Could you check a few things on this model? Use its own coordinates, in mm. A direction names the side the tool comes from. Round coordinates to 2 decimals unless told otherwise and drop trailing zeros. Loops run counter-clockwise (first coordinate to the right, second up) from the corner with the lowest first, then second, coordinate; pieces in that order, holes last.
from build123d import *

# Parameters (mm, degrees)
BASE_FLANGE1_DEPTH = 1000
CUT_EXTRUDE2_DEPTH = 1001.734230453
FILLET1_R          = 5


# Sheet-metal steps are written as plain solids
with BuildPart() as part:
    # Sketch1 → Base-Flange1 (new body)
    with BuildSketch(Plane.XY):
        with BuildLine():
            Line((-35.5, -5), (34.7634, -5))
            ThreePointArc((34.7634, -5), (35.284254855, -4.784254855), (35.5, -4.2634))
            Line((35.5, -4.2634), (35.5, 5))
            Line((35.5, 5), (37, 5))
            Line((37, 5), (37, -4.2634))
            ThreePointArc((37, -4.2634), (36.344915027, -5.844915027), (34.7634, -6.5))
            Line((34.7634, -6.5), (-35.5, -6.5))
            Line((-35.5, -6.5), (-35.5, -5))
        make_face()
    extrude(amount=BASE_FLANGE1_DEPTH)

    # Sketch4 → Cut-Extrude2 (cut, through all)
    with BuildSketch(Plane(origin=(0, -5, 0), x_dir=(1, 0, 0), z_dir=(0, 1, 0))):
        with BuildLine():
            ThreePointArc((-20.5, -62.55), (-23.05, -60), (-20.5, -57.45))
            Line((-20.5, -57.45), (-5.5, -57.45))
            ThreePointArc((-5.5, -57.45), (-2.95, -60), (-5.5, -62.55))
            Line((-5.5, -62.55), (-20.5, -62.55))
        make_face()
        with BuildLine():
            ThreePointArc((-20.5, -602.55), (-23.05, -600), (-20.5, -597.45))
            Line((-20.5, -597.45), (-5.5, -597.45))
            ThreePointArc((-5.5, -597.45), (-2.95, -600), (-5.5, -602.55))
            Line((-5.5, -602.55), (-20.5, -602.55))
        make_face()
        with BuildLine():
            ThreePointArc((-5.5, -937.45), (-2.95, -940), (-5.5, -942.55))
            Line((-5.5, -942.55), (-20.5, -942.55))
            ThreePointArc((-20.5, -942.55), (-23.05, -940), (-20.5, -937.45))
            Line((-20.5, -937.45), (-5.5, -937.45))
        make_face()
        with BuildLine():
            ThreePointArc((-5.5, -397.45), (-2.95, -400), (-5.5, -402.55))
            Line((-5.5, -402.55), (-20.5, -402.55))
            ThreePointArc((-20.5, -402.55), (-23.05, -400), (-20.5, -397.45))
            Line((-20.5, -397.45), (-5.5, -397.45))
        make_face()
    extrude(amount=-CUT_EXTRUDE2_DEPTH, mode=Mode.SUBTRACT)

    # Fillet1
    fillet1_edges = [part.edges().sort_by_distance(p)[0] for p in [
        (-35.5, -5.75, 1000),
        (36.25, 5, 1000),
        (-35.5, -5.75, 0),
        (36.25, 5, 0),
    ]]
    fillet(fillet1_edges, radius=FILLET1_R)


solid = part.part
Item 1: If we section it at A-A, the plane z = 478: Please give me the cut outline in (x, y), then the cut area to 3 significant figures.
Results list:
outline: (-35.5, -6.5) - (34.76, -6.5) arc R2.24 ccw to (37, -4.26) - (37, 5) - (35.5, 5) - (35.5, -4.26) arc R0.74 cw to (34.76, -5) - (-35.5, -5) - close
area: 123 mm2
Item 2: Will these pins go through, and if not, where does the flat tip stop? pin 1 (2 mm diameter, centred on y = -0.5, z = 646.5, fed in from -X); pin 2 (6 mm diameter, centred on x = 29.5, z = 338.5, fed in from +Y).
Results list:
pin 1: stops at x = 35.5
pin 2: stops at y = -5
Item 3: If I drill on line 1 along Z through (x, y) = (-13, -5.25); line 2 along X through (y, z) = (3.75, 712); line 3 along Y through (x, z) = (16, 485.5), over which ranges is the centre line in solid material (lowest first)?
Results list:
line 1: z = 0 to 57.45, 62.55 to 397.45, 402.55 to 597.45, 602.55 to 937.45, 942.55 to 1000
line 2: x = 35.5 to 37
line 3: y = -6.5 to -5
Item 4: For faces 1 (the flat face through (0, -6.5, 493)), 2 (the flat face through (-1, -5, 493)), which set-ups out of +Z, -Z, +X, -X, +Y, -Y let a thin tool reach every point of the face, with its end or its side?
Results list:
face 1: +Z, -Z, +X, -X, -Y
face 2: +Z, -Z, -X, +Y
